from build123d import *

# Parameters (mm, degrees)
SKETCH_R     = 2.6
PAD_DEPTH    = 10
SKETCH002_W  = 6
SKETCH002_H  = 19.473974
POCKET_DEPTH = 18


with BuildPart() as part:
    # Sketch → Pad (new body)
    with BuildSketch(Plane.XZ):
        with BuildLine():
            ThreePointArc((-38.238064, 14.705479), (0, 2.5), (38.238064, 14.705479))
            ThreePointArc((49.277108, 8.519541), (45.715556, 15.106581), (38.238064, 14.705479))
            Line((49.277108, 8.519541), (48.69097, 0))
            Line((-48.69097, 0), (48.69097, 0))
            Line((-49.277108, 8.519541), (-48.69097, 0))
            ThreePointArc((-38.238064, 14.705479), (-45.715556, 15.106581), (-49.277108, 8.519541))
        make_face()
        with Locations((-42.293617, 9)):
            Circle(SKETCH_R, mode=Mode.SUBTRACT)
        with Locations((42.293617, 9)):
            Circle(SKETCH_R, mode=Mode.SUBTRACT)
    extrude(amount=PAD_DEPTH)

    # Sketch002 (on DatumPlane) → Pocket (cut)
    with BuildSketch(Plane.YZ.offset(50)):
        with Locations((-5, 8.823125)):
            Rectangle(SKETCH002_W, SKETCH002_H)
    pocket = extrude(amount=-POCKET_DEPTH, mode=Mode.SUBTRACT)

    # Mirrored: Pocket across YZ
    add(pocket.mirror(Plane.YZ), mode=Mode.SUBTRACT)


solid = part.part
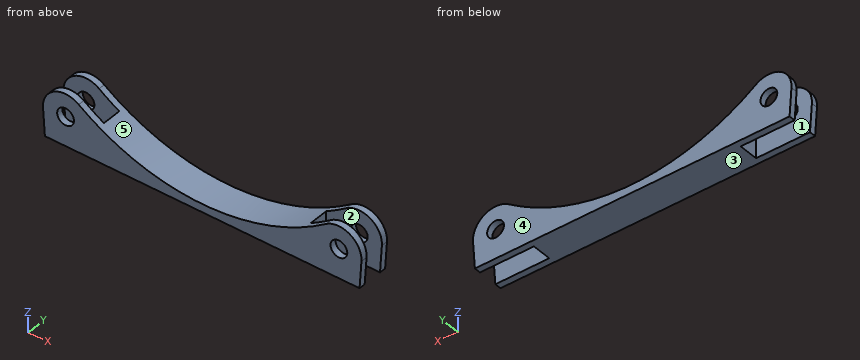
Source: CAD feature listing. Evaluate the final solid. Frame: model axes, mm. Face numbers are marked on the shaded views. A direction names the side the tool comes from. Give positions to 0.01 mm unless a question says otherwise; leave off trailing zeros. Write each loop counter-clockwise with the first axis right and the second up, starting at its lowest first coordinate (ties: lowest second). Pieces come first, ordered by that corner, then holes. Notation, with made-up numbers: M 50.25,-16 L 69.25,-16 A25 cw 69.25,20 Z; hole C -14.5,45 d5. An arc over 180 degrees is marked long. Return JSON: item names as keys, results as strings. Group by question number.
1) Ray query, L1, parallel to Y at x = -37, z = 10.25; L2, parallel to X at y = -0.5, z = 9; L3, parallel to X at y = -0.75, z = 13.75. Return the intervals inside material, ascending.
2) Set-up query: the marked faces 1, 2 and 3. Return all of +Z, -Z, +X, -X, +Y, -Y with unobstructed straight access to the full face (end or side cutting, diameter ignored); none if empty.
3) First-contact query: pin 1 Ø1.5 at (x, y) = (-6.5, -2.5) entering from +Z; pin 2 Ø5 at (x, y) = (-39.5, -3.5) entering from +Z; pin 3 Ø4.5 at (x, z) = (-42.29, 9) entering from -Y; pin 4 Ø5 at (y, z) = (-6, 5.5) entering from +X. Flat tips, straight axial feed; report the tip coordinate or a pass-through.
4) Cut plane D-D, the plane y = -6.75. Output: boundary loops of the cut face in (x, z).
5) Draft query along X for the marked faces 4 and 5. Return one class per face: released by +X, released by -X, zero draft, split by the parting line, or undercut.
6) Cut plane A-A, the plane y = -1. Output: boundary loops of the cut face in (x, z).
7) Cut plane C-C, the plane x = 34.5. Output: boundary loops of the cut face in (y, z) (3 decimals).
8) Cut plane B-B, the plane z = 7.5. Give the number of separate pieces and of enclosed holes in the cut face, then the cut area to 3 significant figures.
Data:
{
 "1": {"L1": "y = -10 to -8, -2 to 0", "L2": "x = -49.29 to -44.89, -39.69 to -28.56, 28.56 to 39.69, 44.89 to 49.29", "L3": "x = -47.44 to -36.86, 36.86 to 47.44"},
 "2": {"face 1": "+Z, -Z, -X", "face 2": "+Z, -Z, +X", "face 3": "-Z, +X, -X, +Y, -Y"},
 "3": {"pin 1": "stops at z = 2.9", "pin 2": "stops at z = 15.95", "pin 3": "passes through", "pin 4": "stops at x = 49.17"},
 "4": {"outline": "M -32,0 L 32,0 L 32,10.78 A66 cw -32,10.78 Z"},
 "5": {"face 4": "zero draft", "face 5": "undercut"},
 "6": {"outline": "M -49.28,8.52 L -48.69,0 L 48.69,0 L 49.28,8.52 A7 ccw 38.24,14.71 A66 cw -38.24,14.71 A7 ccw Z; hole C -42.29,9 d5.2; hole C 42.29,9 d5.2"},
 "7": {"outline": "M -10,0 L -8,0 L -8,12.235 L -10,12.235 Z; M -2,0 L 0,0 L 0,12.235 L -2,12.235 Z"},
 "8": {"separate pieces": "6", "enclosed holes": "0", "area": "240 mm²"}
}
